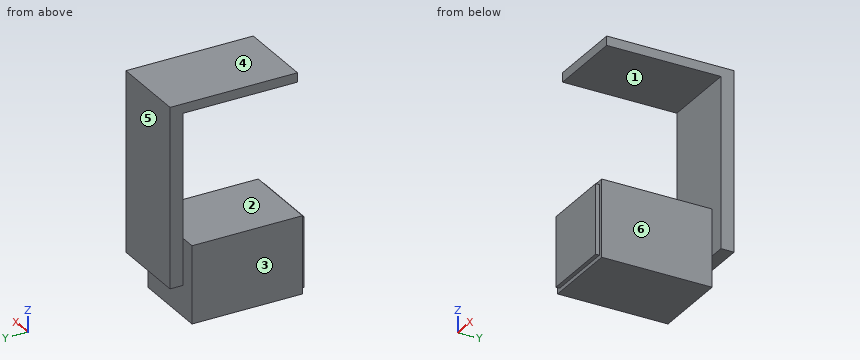
```python
from build123d import *

# Parameters (mm, degrees)
BOSS_EXTRUDE1_DEPTH = 250
SKETCH3_W           = 450
SKETCH3_H           = 450
BOSS_EXTRUDE2_DEPTH = 740
BOSS_EXTRUDE3_START = 25
SKETCH3_3_W         = 500
SKETCH3_3_H         = 500
SKETCH3_3_W_2       = 450
SKETCH3_3_H_2       = 450
BOSS_EXTRUDE3_DEPTH = 715
SKETCH4_W           = 500
SKETCH4_H           = 1160
BOSS_EXTRUDE4_DEPTH = 25


with BuildPart() as part:
    # Sketch2 → Boss-Extrude1 (new, symmetric)
    with BuildSketch(Plane(origin=(0, 0, 0), x_dir=(0, 0, -1), z_dir=(1, 0, 0))):
        Polygon((0, 0), (0, 800), (1160, 800), (1160, 740), (60, 740), (60, 0), align=None)
    extrude(amount=BOSS_EXTRUDE1_DEPTH, both=True)

    # Sketch3 → Boss-Extrude2 (add)
    with BuildSketch(Plane(origin=(0, 0, 0), x_dir=(1, 0, 0), z_dir=(0, 1, 0))):
        with Locations((-100, 1110)):
            Rectangle(SKETCH3_W, SKETCH3_H)
    extrude(amount=BOSS_EXTRUDE2_DEPTH)

    # Sketch3<3> → Boss-Extrude3 (add)
    with BuildSketch(Plane(origin=(0, 0, 0), x_dir=(1, 0, 0), z_dir=(0, 1, 0)).offset(BOSS_EXTRUDE3_START)):
        with Locations((-100, 1110)):
            Rectangle(SKETCH3_3_W, SKETCH3_3_H)
        with Locations((-100, 1110)):
            Rectangle(SKETCH3_3_W_2, SKETCH3_3_H_2, mode=Mode.SUBTRACT)
    extrude(amount=BOSS_EXTRUDE3_DEPTH)

    # Sketch4 → Boss-Extrude4 (add)
    with BuildSketch(Plane(origin=(0, 800, 0), x_dir=(1, 0, 0), z_dir=(0, 1, 0))):
        with Locations((0, 580)):
            Rectangle(SKETCH4_W, SKETCH4_H)
    extrude(amount=BOSS_EXTRUDE4_DEPTH)


solid = part.part
```
Check sheet for the modelled part. Datum: model origin and axes. Units: mm. Face numbers are marked on the shaded views. A direction names the side the tool comes from. Coordinates: 2 decimals unless noted, no trailing zeros. Order: outer loops, then holes, each group sorted by start corner. A loop starts at its lowest first (then second) coordinate and runs counter-clockwise, first axis right, second up. Notation, with made-up numbers: M 24.25,79 L 41.25,79 A15 cw 41.25,99 Z; hole C 10,3.5 d10. An arc over 180 degrees is marked long. One line per question, with ' | ' between items. Start each with the question number.
Item 1: Sectioned sample at D-D on x = 195.5. Record the cut outline in (y, z).
Item 2: Sectioned sample at A-A on y = 580.5. Record the cut outline in (x, z).
Item 3: Sectioned sample at C-C on z = -1081. Record the cut outline in (x, y), and give its area (3 significant figures).
Item 4: Gauge pin test, flat ends, axial feed: P1, Ø20, axis at x = -182.5, y = 10, coming from the -Z side; P2, Ø20, axis at y = 14.5, z = -1202, coming from the +X side; P3, Ø2, axis at x = 147.5, z = -251.5, coming from the -Y side. Record the tip position at first contact, or that the pin passes through.
Item 5: Access from +Z, -Z, +X, -X, +Y, -Y to the whole of each face (thin tool, end or side, straight path). Record for the marked faces 5 and 6.
Item 6: Material ranges on line 1 (Z direction, x = 35, y = 120); line 2 (Y direction, x = -15.5, z = -185); line 3 (Z direction, x = 193, y = 621), recorded low to high.
Item 7: Sectioned sample at B-B on x = 54.5. Record the cut outline in (y, z).
Item 8: Mould release check, pull along Z, two halves, no side actions. Record for the marked faces 1, 2, 3 and 4: pulls with the +Z half, pulls with the -Z half, needs draft (parallel to the pull), parting line crosses it, or undercut.
Answer below:
1) outline: M 0,-60 L 740,-60 L 740,-1160 L 825,-1160 L 825,0 L 0,0 Z
2) outline: M -350,-1360 L 150,-1360 L 150,-860 L -350,-860 Z; M -250,-60 L 250,-60 L 250,0 L -250,0 Z
3) outline: M -350,25 L -325,25 L -325,0 L 125,0 L 125,25 L 150,25 L 150,740 L 250,740 L 250,825 L -250,825 L -250,740 L -350,740 Z | area: 411,000 mm^2
4) P1: stops at z = -1335 | P2: stops at x = 125 | P3: stops at y = 740
5) face 5: +Z, -Z, +X, -X, +Y | face 6: -Z, +X, -Y
6) line 1: z = -1360 to -860, -60 to 0 | line 2: y = 740 to 825 | line 3: z = -60 to 0
7) outline: M 0,-1335 L 25,-1335 L 25,-1360 L 740,-1360 L 740,-1160 L 825,-1160 L 825,0 L 0,0 L 0,-60 L 740,-60 L 740,-860 L 25,-860 L 25,-885 L 0,-885 Z
8) face 1: undercut | face 2: undercut | face 3: needs draft | face 4: pulls with the +Z half
